Source: CAD feature listing. Evaluate the final solid. Frame: model axes, mm. Face numbers are marked on the shaded views. A direction names the side the tool comes from. Give positions to 0.01 mm unless a question says otherwise; leave off trailing zeros. Write each loop counter-clockwise with the first axis right and the second up, starting at its lowest first coordinate (ties: lowest second). Pieces come first, ordered by that corner, then holes. Notation, with made-up numbers: M 1.25,45 L 27.25,45 A35 ccw 27.25,80 Z; hole C 46.25,-23 d6. An arc over 180 degrees is marked long. Use CSV: the item, a comma, the result in double quotes. Start each with the question number.
from build123d import *

# Parameters (mm, degrees)
F1_DEPTH = 120
F3_DEPTH = 5
F5_D     = 6.6
F5_DEPTH = 14.4
F5_TIP   = 1.9828400428


with BuildPart() as f1:
    # F0 (on Right) → F1 (new body, symmetric)
    with BuildSketch(Plane.YZ):
        Polygon((5, 250), (0, 250), (0, 0), (65, 0), (65, 5), (5, 5), align=None)
    extrude(amount=F1_DEPTH, both=True)

    # F2 (on face) → F3 (cut, through all)
    with BuildSketch(Plane(origin=(0, 5, 0), x_dir=(-1, 0, 0), z_dir=(0, 1, 0))):
        with BuildLine():
            ThreePointArc((-42, 154), (0, 112), (42, 154))
            Line((42, 154), (42, 250))
            Line((42, 250), (-42, 250))
            Line((-42, 250), (-42, 154))
        make_face()
    extrude(amount=-F3_DEPTH, mode=Mode.SUBTRACT)

    # F5
    with Locations(Plane.XY.offset(5)):
        with Locations((-100, 20), (-100, 50), (100, 20), (100, 50)):
            Hole(F5_D / 2, depth=F5_DEPTH)
            with Locations((0, 0, -(F5_DEPTH + F5_TIP / 2))):  # 118° drill point
                Cone(0, F5_D / 2, F5_TIP, mode=Mode.SUBTRACT)


solid = f1.part
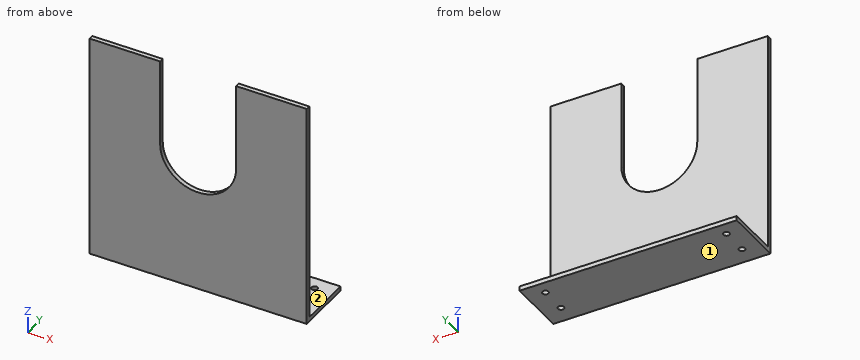
1. Section B-B on z = 216. Return loops of the section in (x, y).
2. Section D-D on x = 52.5. Return loops of the section in (y, z).
3. Line query: probe 1 along Y at (x, z) = (100, 2); probe 2 along Z at (x, y) = (79, 44). Output: solid intervals per line, ascending.
4. Access query for the marked faces 1 and 2. Directions: +Z, -Z, +X, -X, +Y, -Y. A direction counts if a zero-diameter tool reaches every point of the face in a straight line with its end or side. Return the directions, or none.
5. Section C-C on y = 20. Return loops of the section in (x, z).
6. First-contact query: pin 1 (10 mm diameter, centred on x = -41.5, y = 19.5, fed in from +Z); pin 2 (10.5 mm diameter, centred on x = 100, y = 50, fed in from -Z); pin 3 (1 mm diameter, centred on x = -22, z = 113, fed in from +Y); pin 4 (4 mm diameter, centred on x = -100, y = 50, fed in from +Z). Flat tips, straight axial feed; report the tip coordinate or a pass-through.
7. Section A-A on x = -100. Return loops of the section in (y, z), then the cut area to 3 significant figures.
Resolved:
1,outline,"M -120,0 L -42,0 L -42,5 L -120,5 Z; M 42,0 L 120,0 L 120,5 L 42,5 Z"
2,outline,"M 0,0 L 65,0 L 65,5 L 5,5 L 5,250 L 0,250 Z"
3,probe 1,"y = 0 to 16.7, 23.3 to 46.7, 53.3 to 65"
3,probe 2,"z = 0 to 5"
4,face 1,"-Z, +X, -X, +Y, -Y"
4,face 2,"+Z, +X, -X, +Y"
5,outline,"M -120,0 L -103.3,0 L -103.3,5 L -120,5 Z; M -96.7,0 L 96.7,0 L 96.7,5 L -96.7,5 Z; M 103.3,0 L 120,0 L 120,5 L 103.3,5 Z"
6,pin 1,"stops at z = 5"
6,pin 2,"stops at z = 0"
6,pin 3,"stops at y = 5"
6,pin 4,"passes through"
7,outline,"M 0,0 L 16.7,0 L 16.7,5 L 5,5 L 5,250 L 0,250 Z; M 23.3,0 L 46.7,0 L 46.7,5 L 23.3,5 Z; M 53.3,0 L 65,0 L 65,5 L 53.3,5 Z"
7,area,"1,480 mm2"
